Answer from the drawing. Dimensions are ordinates in mm from the lowest x, y and z of the part. A direction names the side the tool comes from. Coordinates: 2 decimals unless noted, no trailing zeros. Write each loop counter-clockwise with the first axis right and the second up, starting at its lowest first coordinate (ties: lowest second). Pieces come first, ordered by that corner, then holes.
(1) Section D-D on x = 3 is taken. Write down the section's boundary in (y, z), then the cut area to 3 significant figures.
(2) Given pin 1 (2 mm diameter, centred on x = 8.5, y = 4, fed in from +Z); pin 2 (6 mm diameter, centred on y = 3.5, z = 8, fed in from -X); pin 3 (0.9 mm diameter, centred on x = 2.5, y = 5, fed in from +Z), each flat-ended and moving along its own axis, determine where each tip first touches the part or whether it passes through.
(3) Section A-A on z = 18 is taken. Write down the section's boundary in (x, y), then the cut area to 3 significant figures.
(4) Section B-B on y = 5 is taken. Write down the section's boundary in (x, z), then the cut area to 3 significant figures.
(5) Which of the six approach directions +Z, -Z, +X, -X, +Y, -Y give full straight-line access (tool end or side, diameter ignored) to the marked faces 4, 5 and 6?
(6) Find the intervals of material crossed by probe 1 along Z at (x, y) = (11.9, 5); probe 2 along Z at (x, y) = (9.5, 0.5); probe 3 along X at (y, z) = (5.25, 13.75), in increasing order.
(7) The mould has two halves that part along Y. Classify the marked faces 1, 2 and 3: +Y half, -Y half, draft (parallel to the pull), parting line (faces both ways), or undercut.
(8) Section C-C on x = 12 is taken. Write down the section's boundary in (y, z), then the cut area to 3 significant figures.
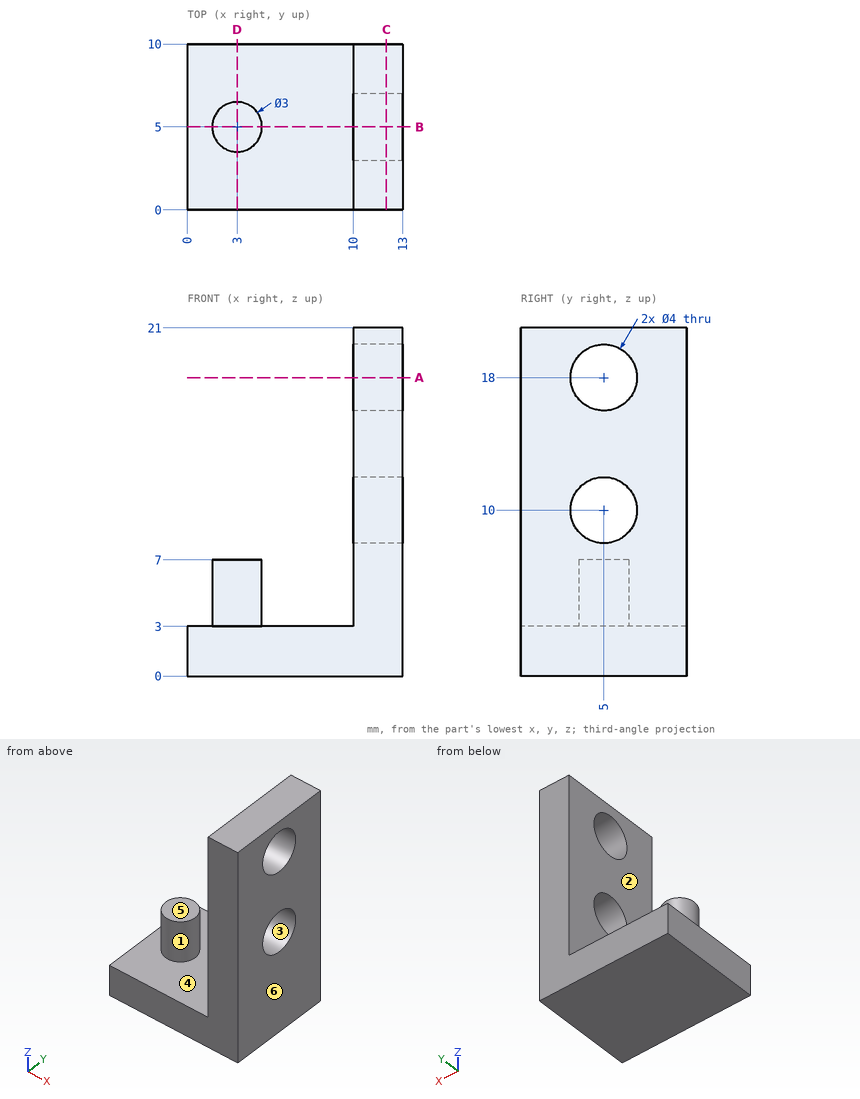
Response:
1. outline: (0, 0) - (10, 0) - (10, 3) - (6.5, 3) - (6.5, 7) - (3.5, 7) - (3.5, 3) - (0, 3) - close
1. area: 42.0 mm2
2. pin 1: stops at z = 3
2. pin 2: stops at x = 1.5
2. pin 3: stops at z = 7
3. outline: (10, 0) - (13, 0) - (13, 3) - (10, 3) - close; (10, 7) - (13, 7) - (13, 10) - (10, 10) - close
3. area: 18.0 mm2
4. outline: (0, 0) - (13, 0) - (13, 8) - (10, 8) - (10, 3) - (4.5, 3) - (4.5, 7) - (1.5, 7) - (1.5, 3) - (0, 3) - close; (10, 12) - (13, 12) - (13, 16) - (10, 16) - close; (10, 20) - (13, 20) - (13, 21) - (10, 21) - close
4. area: 81.0 mm2
5. face 4: +Z
5. face 5: +Z, -X, +Y, -Y
5. face 6: +Z, -Z, +X, +Y, -Y
6. probe 1: z = 0 to 8, 12 to 16, 20 to 21
6. probe 2: z = 0 to 3
6. probe 3: x = 10 to 13
7. face 1: parting line
7. face 2: draft
7. face 3: undercut
8. outline: (0, 0) - (10, 0) - (10, 21) - (0, 21) - close; hole circle Ø4 at (5, 10); hole circle Ø4 at (5, 18)
8. area: 185 mm2
